Autodesk Inventor part; units mm, degrees
ref_plane "YZ Plane" through (0, 0, 0) normal (1, 0, 0) x (0, 1, 0)
ref_plane "XZ Plane" through (0, 0, 0) normal (0, 1, 0) x (-1, 0, 0)
ref_plane "XY Plane" through (0, 0, 0) normal (0, 0, 1) x (1, 0, 0)
sketch "スケッチ1" plane through (0, 0, 0) normal (0, 0, 1) x (1, 0, 0)
  circle A0 centre (0, 0) radius 1.5
  circle A1 centre (0, 0) radius 10.5
  dimension "d0" = 3
  dimension "d1" = 21
extrude "押し出し1" add sketch "スケッチ1" along normal blind 2
sketch "スケッチ2" plane through (0, 0, 2) normal (0, 0, 1) x (1, 0, 0)
  circle A0 centre (0, 0) radius 10.5
  circle A1 centre (0, 0) radius 1.5
  circle A2 centre (0, 0) radius 8
  circle A3 centre (0, 0) radius 4
  dimension "d4" = 2.5
  dimension "d5" = 2.5
  dimension "d6" = 4
extrude "押し出し2" cut sketch "スケッチ2" against normal blind 1.3 contours A2
properties part number "ウィング引っ掛け" material "ポリカーボネート、スモーク"
Geometry check sheet. Reference: the model listing, model coordinates, mm. A direction names the side the tool comes from. Round coordinates to 2 decimals unless told otherwise and drop trailing zeros. Loops run counter-clockwise (first coordinate to the right, second up) from the corner with the lowest first, then second, coordinate; pieces in that order, holes last. Notation, with made-up numbers: (70, 68.25) -> (117, 68.25) arc R30 ccw to (117, 92.25) -> close; hole circle Ø10 at (-12.75, 14). An arc over 180 degrees is marked (long way). Answer as a JSON object with one key per item and string values. Group by question number.
Item 1: Cross-section at A-A, the plane x = 0. Record the cut outline in (y, z).
Item 2: Release check for a two-part mould opening along Y. For faces 3 (the face through (10, -3.2, 1)), 4 (the face through (-2, -8, 2)), 5 (the face through (-1.73, -7.81, 1.36)) record: pulls with the +Y half, pulls with the -Y half, needs draft (parallel to the pull), parting line crosses it, or undercut.
Item 3: Depth check by flat-ended pin: pin 1 Ø2 at (x, y) = (5, 5) entering from +Z; pin 2 Ø1.8 at (x, y) = (0, 0) entering from -Z; pin 3 Ø1 at (x, z) = (4, 1) entering from -Y. Enter the tip coordinate at first touch or a pass-through.
Item 4: Set-up check for faces 1 (the face through (-0.867, -3.905, 1.359)), 2 (the face through (2, 0, 0)): record each of +Z, -Z, +X, -X, +Y, -Y from which the full face is reachable in a straight line by a thin tool's end or side.
Item 5: Cross-section at C-C, the plane z = 1.75. Record the cut outline in (x, y), plus the area to 3 significant figures.
Item 6: Cross-section at D-D, the plane x = 3.5. Record the cut outline in (y, z), plus the area to 3 significant figures.
Item 7: Thickness scan on line 1 along Y through (x, z) = (0, 1.45); line 2 along Z through (x, y) = (7.5, 1.75); line 3 along X through (y, z) = (6.5, 1.55). Record the ranges inside material, lowest first.
Determined:
{
 "1": {"outline": "(-10.5, 0) -> (-1.5, 0) -> (-1.5, 2) -> (-4, 2) -> (-4, 0.7) -> (-8, 0.7) -> (-8, 2) -> (-10.5, 2) -> close; (1.5, 0) -> (10.5, 0) -> (10.5, 2) -> (8, 2) -> (8, 0.7) -> (4, 0.7) -> (4, 2) -> (1.5, 2) -> close"},
 "2": {"face 3": "parting line crosses it", "face 4": "needs draft", "face 5": "undercut"},
 "3": {"pin 1": "stops at z = 2", "pin 2": "passes through", "pin 3": "stops at y = -9.9"},
 "4": {"face 1": "+Z", "face 2": "-Z, +X, -X, +Y, -Y"},
 "5": {"outline": "circle Ø21 at (0, 0); circle Ø8 at (0, 0); hole circle Ø16 at (0, 0); hole circle Ø3 at (0, 0)", "area": "188 mm²"},
 "6": {"outline": "(-9.9, 0) -> (9.9, 0) -> (9.9, 2) -> (7.19, 2) -> (7.19, 0.7) -> (1.94, 0.7) -> (1.94, 2) -> (-1.94, 2) -> (-1.94, 0.7) -> (-7.19, 0.7) -> (-7.19, 2) -> (-9.9, 2) -> close", "area": "25.9 mm²"},
 "7": {"line 1": "y = -10.5 to -8, -4 to -1.5, 1.5 to 4, 8 to 10.5", "line 2": "z = 0 to 0.7", "line 3": "x = -8.25 to -4.66, 4.66 to 8.25"}
}
